For this review, use the dimensioned drawing (mm, ordinates from the lowest corner) and the shaded views. A direction names the side the tool comes from. Coordinates: 2 decimals unless noted, no trailing zeros. Write each loop counter-clockwise with the first axis right and the second up, starting at its lowest first coordinate (ties: lowest second). Pieces come first, ordered by that corner, then holes. Notation, with made-up numbers: M 60,-25 L 64,-25 A20 cw 64,-7 Z; hole C 65,25.5 d9. An arc over 180 degrees is marked long. One line per question, with ' | ' between items.
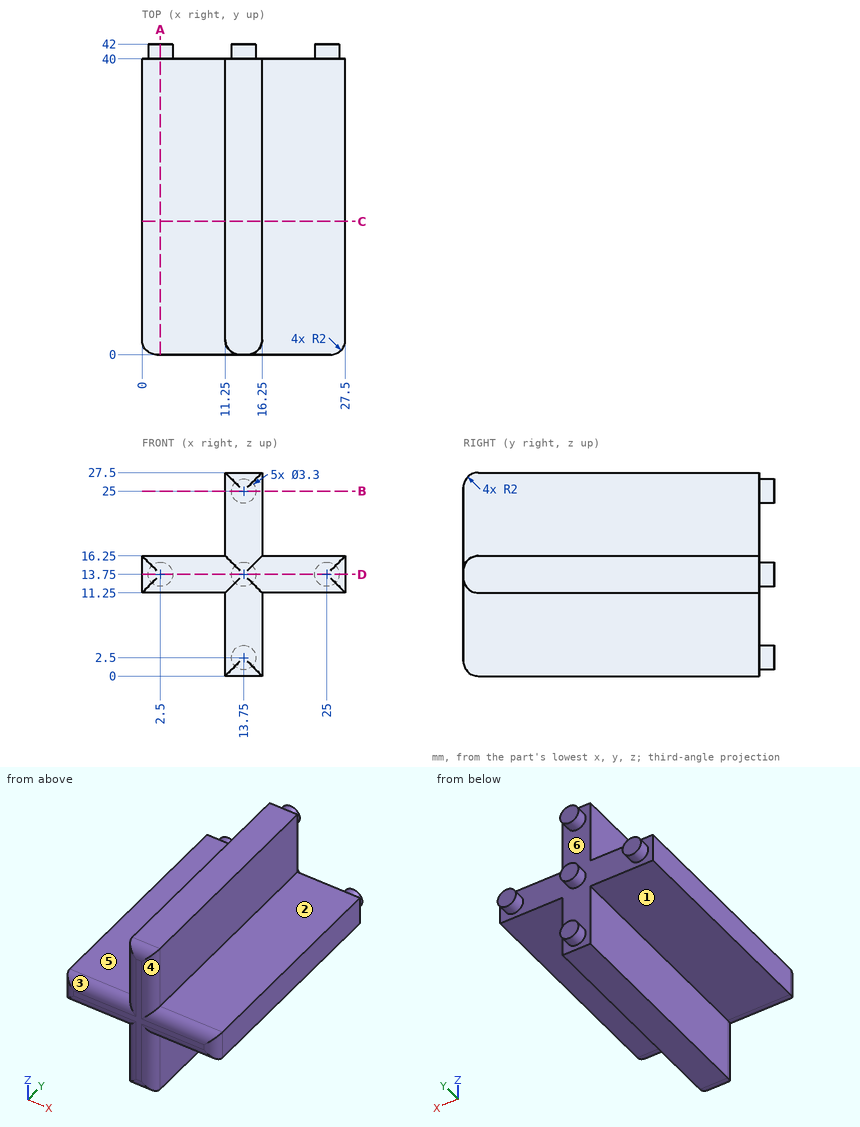
1) To check wall thickness, follow line 1 along Z through (x, y) = (20.25, 38.5); line 2 along Y through (x, z) = (15, 2). State the ranges of each line that lie inside material, in increasing order. Write a range as [from, to].
Responses:
line 1: [11.25, 16.25] | line 2: [0.15, 42]
2) Insertion check: pin 1 Ø12.5 at (x, y) = (23.5, 29) entering from -Z; pin 2 Ø3.5 at (x, y) = (19.5, 23.5) entering from +Z; pin 3 Ø3.5 at (y, z) = (26, 6) entering from -X. Each pin has a flat end and moves straight along its axis. Give the tip position at first contact, or say it passes through.
Responses:
pin 1: z = 11.25 | pin 2: z = 16.25 | pin 3: x = 11.25
3) The part is to be moulded in two halves that separate along Z. For the marked faces 4, 5 and 6, say which applies: +Z half, -Z half, draft (parallel to the pull), parting line (faces both ways), or undercut.
Responses:
face 4: draft | face 5: +Z half | face 6: undercut
4) We need section A-A on x = 2.5. State the section outline as (y, z) points, then the cut area to 3 significant figures.
Responses:
outline: M 0,13.25 A2 ccw 2,11.25 L 40,11.25 L 40,12.1 L 42,12.1 L 42,15.4 L 40,15.4 L 40,16.25 L 2,16.25 A2 ccw 0,14.25 Z | area: 205 mm^2
5) We need section C-C on y = 18. State the section outline as (x, z) points.
Responses:
outline: M 0,11.25 L 11.25,11.25 L 11.25,0 L 16.25,0 L 16.25,11.25 L 27.5,11.25 L 27.5,16.25 L 16.25,16.25 L 16.25,27.5 L 11.25,27.5 L 11.25,16.25 L 0,16.25 Z
6) We need section D-D on z = 13.75. State the section outline as (x, y) points.
Responses:
outline: M 0,2 A2 ccw 2,0 L 25.5,0 A2 ccw 27.5,2 L 27.5,40 L 26.65,40 L 26.65,42 L 23.35,42 L 23.35,40 L 15.4,40 L 15.4,42 L 12.1,42 L 12.1,40 L 4.15,40 L 4.15,42 L 0.85,42 L 0.85,40 L 0,40 Z
7) Machinability: for the marked faces 1, 2 and 3, which of the approach directions +Z, -Z, +X, -X, +Y, -Y give a long, thin tool a straight path to every point of the face, cutting with its end or side? Answer none if there is none.
Responses:
face 1: -Z, -X, +Y, -Y | face 2: +Z, +X, +Y, -Y | face 3: +Z, -X, -Y
8) We need section B-B on z = 25. State the section outline as (x, y) points, then the cut area to 3 significant figures.
Responses:
outline: M 11.25,2 A2 ccw 13.25,0 L 14.25,0 A2 ccw 16.25,2 L 16.25,40 L 15.4,40 L 15.4,42 L 12.1,42 L 12.1,40 L 11.25,40 Z | area: 205 mm^2
